Part print with two shaded views. Sizes in mm from the minimum x, y, z corner. A direction names the side the tool comes from. Give positions to 0.01 mm unless a question says otherwise; leave off trailing zeros. Order: outer loops, then holes, each group sorted by start corner. A loop starts at its lowest first (then second) coordinate and runs counter-clockwise, first axis right, second up. Notation, with made-up numbers: M -18.5,50.5 L 34.5,50.5 A18 ccw 34.5,59.5 Z; hole C -4,41.5 d10. An arc over 180 degrees is marked long. Return JSON: item names as keys, results as strings.
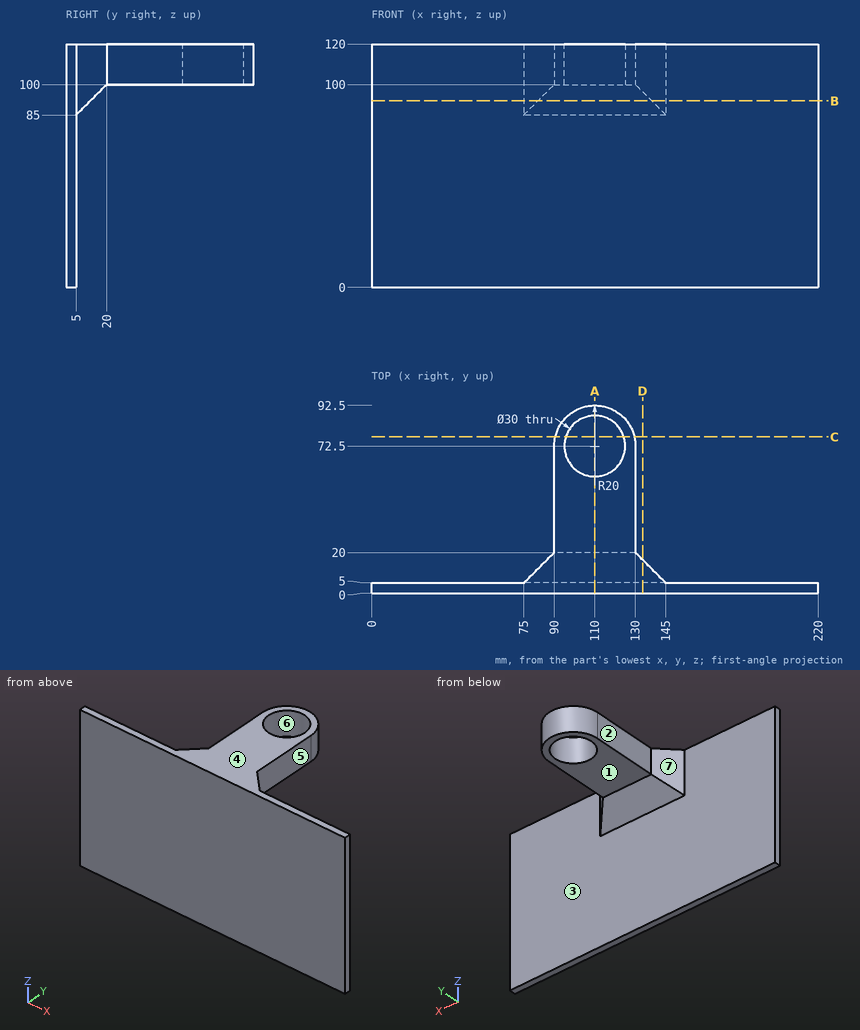
Q1. Band-saw the part on D-D (x = 133.5). Give the cut face in (y, z), then the cut area to 3 significant figures.
Established:
{"outline": "M 0,0 L 5,0 L 5,85 L 16.5,96.5 L 16.5,120 L 0,120 Z", "area": "936 mm²"}
Q2. Pin check, flat tips, straight feed: pin 1 (4 mm diameter, centred on x = 196, z = 103.5, fed in from +Y); pin 2 (10 mm diameter, centred on y = 47.5, z = 108.5, fed in from -X); pin 3 (6 mm diameter, centred on x = 121.5, z = 91, fed in from +Y). Stop position of each tip, or through.
Established:
{"pin 1": "stops at y = 5", "pin 2": "stops at x = 90", "pin 3": "stops at y = 14"}
Q3. Band-saw the part on A-A (x = 110). Give the cut face in (y, z), then the cut area to 3 significant figures.
Established:
{"outline": "M 0,0 L 5,0 L 5,85 L 20,100 L 57.5,100 L 57.5,120 L 0,120 Z; M 87.5,100 L 92.5,100 L 92.5,120 L 87.5,120 Z", "area": "1,860 mm²"}
Q4. Two-plate mould, pull along X, no slides. Class the marked faces 5, 6 and 7: +X half, -X half, draft (parallel to the pull), parting line (faces both ways), or undercut.
Established:
{"face 5": "+X half", "face 6": "undercut", "face 7": "-X half"}
Q5. Band-saw the part on C-C (y = 77). Give the cut face in (x, z), then the cut area to 3 significant figures.
Established:
{"outline": "M 90.51,100 L 95.69,100 L 95.69,120 L 90.51,120 Z; M 124.31,100 L 129.49,100 L 129.49,120 L 124.31,120 Z", "area": "207 mm²"}
Q6. 3-axis set-ups, long thin cutter, end or side, ignore diameter. For the marked faces 1, 2, 3 and 4: which of +Z, -Z, +X, -X, +Y, -Y reach the whole face in a straight line?
Established:
{"face 1": "-Z, +X, -X, +Y", "face 2": "+Z, -Z, -X, +Y", "face 3": "-Z, +Y", "face 4": "+Z, +X, -X, +Y, -Y"}
Q7. Band-saw the part on B-B (z = 92). Give the cut face in (x, y), then the cut area to 3 significant figures.
Established:
{"outline": "M 0,0 L 220,0 L 220,5 L 145,5 L 138,12 L 82,12 L 75,5 L 0,5 Z", "area": "1,540 mm²"}
Q8. Probe line 1 along Y through (x, z) = (110, 105); line 2 along X through (y, z) = (72, 106); line 3 along Y through (x, z) = (150.5, 20). List the from-to ranges inside material, lowest first.
Established:
{"line 1": "y = 0 to 57.5, 87.5 to 92.5", "line 2": "x = 90 to 95.01, 124.99 to 130", "line 3": "y = 0 to 5"}
